```python
from build123d import *

# Parameters (mm, degrees)
F0_R     = 20
F0_W     = 150
F0_H     = 55
F1_DEPTH = 125


with BuildPart() as f1:
    # F0 (on Top) → F1 (new body, symmetric)
    with BuildSketch(Plane.XY):
        Polygon((27.5, -125), (95, -125), (125, -95), (125, 95), (95, 125), (27.5, 125), (27.5, 75), (-27.5, 75), (-27.5, 125), (-95, 125), (-125, 95), (-125, -95), (-95, -125), (-27.5, -125), (-27.5, -75), (27.5, -75), align=None)
        with Locations((-75, -75)):
            Circle(F0_R, mode=Mode.SUBTRACT)
        with Locations((75, -75)):
            Circle(F0_R, mode=Mode.SUBTRACT)
        with Locations((-75, 75)):
            Circle(F0_R, mode=Mode.SUBTRACT)
        Rectangle(F0_W, F0_H, mode=Mode.SUBTRACT)
        with Locations((75, 75)):
            Circle(F0_R, mode=Mode.SUBTRACT)
    extrude(amount=F1_DEPTH, both=True)


solid = f1.part
```
Geometry check sheet. Reference: the model listing, model coordinates, mm. A direction names the side the tool comes from. Round coordinates to 2 decimals unless told otherwise and drop trailing zeros. Loops run counter-clockwise (first coordinate to the right, second up) from the corner with the lowest first, then second, coordinate; pieces in that order, holes last. Notation, with made-up numbers: (-22, -3.75) - (-8, -3.75) arc R11 ccw to (-8, 17.25) - close; hole circle Ø9 at (4, 15.25). An arc over 180 degrees is marked (long way). Use a Markdown table: item, result.
Q1. Go/stop test with flat-tipped pins: P1, Ø16.5, axis at x = -13.5, z = -46, coming from the -Y side; P2, Ø6, axis at x = 6, z = -61.5, coming from the +Y side. Record where each tip stops, or that it passes through.
Solutions:
| item | result |
|---|---|
| P1 | stops at y = -75 |
| P2 | stops at y = 75 |
Q2. Cross-section at A-A on y = -12. Record the cut outline in (x, z), plus the area to 3 significant figures.
Solutions:
| item | result |
|---|---|
| outline | (-125, -125) - (-75, -125) - (-75, 125) - (-125, 125) - close; (75, -125) - (125, -125) - (125, 125) - (75, 125) - close |
| area | 25,000 mm2 |
Q3. Draft check along Y on faces 6 (the flat face through (27.5, 100, 2)), 7 (the cylindrical face through (-79.336, -94.524, -1.75)), 8 (the flat face through (110, 110, 2)). Enter one of: released by +Y, released by -Y, zero draft, split by the parting line, or undercut.
Solutions:
| item | result |
|---|---|
| face 6 | zero draft |
| face 7 | undercut |
| face 8 | released by +Y |
Q4. Material ranges on line 1 (X direction, y = 12, z = 55.5); line 2 (Y direction, x = -9, z = 32.5); line 3 (Y direction, x = -53, z = 85.5), recorded low to high.
Solutions:
| item | result |
|---|---|
| line 1 | x = -125 to -75, 75 to 125 |
| line 2 | y = -75 to -27.5, 27.5 to 75 |
| line 3 | y = -125 to -27.5, 27.5 to 125 |
Q5. Access from +Z, -Z, +X, -X, +Y, -Y to the whole of each face (thin tool, end or side, straight path). Record for faces 1 (the flat face through (-2, 30, 125)), 2 (the flat face through (0, -75, 2)), 3 (the flat face through (-27.5, 100, 2)), 4 (the flat face through (-1, -27.5, 2)), 5 (the flat face through (-2, 30, -125)).
Solutions:
| item | result |
|---|---|
| face 1 | +Z, +X, -X, +Y, -Y |
| face 2 | +Z, -Z, -Y |
| face 3 | +Z, -Z, +Y |
| face 4 | +Z, -Z |
| face 5 | -Z, +X, -X, +Y, -Y |
Q6. Cross-section at B-B on z = 82. Record the cut outline in (x, y), plus the area to 3 significant figures.
Solutions:
| item | result |
|---|---|
| outline | (-125, -95) - (-95, -125) - (-27.5, -125) - (-27.5, -75) - (27.5, -75) - (27.5, -125) - (95, -125) - (125, -95) - (125, 95) - (95, 125) - (27.5, 125) - (27.5, 75) - (-27.5, 75) - (-27.5, 125) - (-95, 125) - (-125, 95) - close; hole circle Ø40 at (-75, -75); hole circle Ø40 at (-75, 75); hole (-75, -27.5) - (75, -27.5) - (75, 27.5) - (-75, 27.5) - close; hole circle Ø40 at (75, -75); hole circle Ø40 at (75, 75) |
| area | 41,900 mm2 |
Q7. Cross-section at C-C on y = 67. Record the cut outline in (x, z), plus the area to 3 significant figures.
Solutions:
| item | result |
|---|---|
| outline | (-125, -125) - (-93.33, -125) - (-93.33, 125) - (-125, 125) - close; (-56.67, -125) - (56.67, -125) - (56.67, 125) - (-56.67, 125) - close; (93.33, -125) - (125, -125) - (125, 125) - (93.33, 125) - close |
| area | 44,200 mm2 |
